Here's how the part is built. I have some questions about the finished solid (model axes, mm). Face numbers are marked on the shaded views. A direction names the side the tool comes from. Coordinates: 2 decimals unless noted, no trailing zeros. Write each loop counter-clockwise with the first axis right and the second up, starting at its lowest first coordinate (ties: lowest second). Pieces come first, ordered by that corner, then holes. Notation, with made-up numbers: (38.5, 9) -> (67.5, 9) arc R27 ccw to (67.5, 47) -> close; hole circle Ø7 at (80, -5.75). An arc over 180 degrees is marked (long way). Put each result on its own line as item: value.
Autodesk Inventor part; units mm, degrees
ref_plane "YZ Plane" through (0, 0, 0) normal (1, 0, 0) x (0, 1, 0)
ref_plane "XZ Plane" through (0, 0, 0) normal (0, 1, 0) x (-1, 0, 0)
ref_plane "XY Plane" through (0, 0, 0) normal (0, 0, 1) x (1, 0, 0)
sketch "Sketch1" plane through (0, 0, 0) normal (0, 0, 1) x (1, 0, 0)
  line L0 (0, 0) -> (60, 0)
  line L1 (60, 0) -> (60, 24)
  line L2 (60, 24) -> (0, 24)
  line L3 (0, 24) -> (0, 0)
  dimension "d0" = 60
  dimension "d1" = 24
extrude "Extrusion1" add sketch "Sketch1" along normal blind 51.8
sketch "Sketch2" plane through (60, 0, 0) normal (1, 0, 0) x (0, 0, -1)
  line L0 (-51.8, 24) -> (-51.8, 0)
  line L1 (0, 0) -> (-51.8, 0)
  line L2 (0, 0) -> (0, 24)
  line L3 (0, 24) -> (-51.8, 24)
  line L4 (-51.8, 14) -> (-18, 14)
  arc A0 (-18, 6) -> (-6, 6) centre (-12, 6) ccw
  line L5 (-18, 6) -> (-18, 14)
  line L6 (-6, 6) -> (-6, 19)
  line L7 (-6, 19) -> (0, 19)
  dimension "d5" = 10
  dimension "d6" = 18
  dimension "d7" = 12
  dimension "d8" = 5
  dimension "d9" = 6
extrude "Extrusion2" cut sketch "Sketch2" against normal blind 60 contours L4 L5 A0 L1 L0 | L2 L1 A0 L6 L7
sketch "Sketch3" plane through (0, 0, 51.8) normal (0, 0, 1) x (1, 0, 0)
  line L0 (60, 0) -> (0, 0)
  line L1 (55, 19) -> (55, 0)
  line L2 (55, 0) -> (60, 0)
  line L3 (60, 0) -> (60, 19)
  line L4 (5, 19) -> (5, 0)
  line L5 (5, 0) -> (0, 0)
  line L6 (0, 0) -> (0, 19)
  line L7 (60, 19) -> (0, 19)
  line L8 (0, 24) -> (60, 24)
  line L9 (0, 0) -> (0, 24)
  line L10 (60, 24) -> (60, 0)
  line L11 (0, 19) -> (5, 19)
  line L12 (55, 19) -> (60, 19)
  point P0 (0, 14)
  point P1 (60, 14)
  dimension "d16" = 5
  dimension "d17" = 5
extrude "Extrusion3" cut sketch "Sketch3" against normal blind 52 contours L0 L1 L7 L3 | L0 L6 L7 L4
chamfer "Chamfer1" distance 10 angle 15 1 edges at (30, 24, 51.8) measured on face at (21.6667, 22.3333, 51.8)
sketch "Sketch5" plane through (55, 19, 6) normal (0, 0, -1) x (-1, 0, 0)
  line L0 (0, 0) -> (0, -13)
  line L1 (-5, 5) -> (55, 5)
  point P0 (55, -19)
  point P1 (6, -9)
  point P2 (44, -9)
  dimension "d35" = 38
  dimension "d36" = 6
  dimension "d37" = 14
  dimension "d38" = 14
hole "Hole2" at (49, 10, 6) at (11, 10, 6) direction (0, 0, 1) diameter 4.917 depth 10 tip angle 118
chamfer "Chamfer2" distance 0.5 angle 45 2 edges at (11, 7.5415, 6) (49, 7.5415, 6)
properties part number "TETO DA CABINE(15)" material "Carbon Steel"
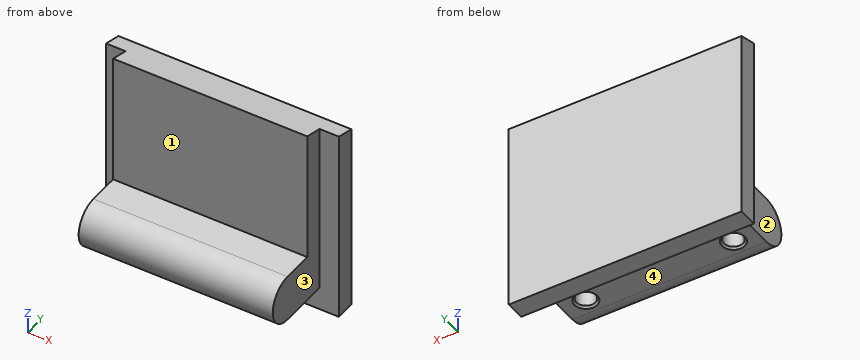
Item 1: Which directions (+Z, -Z, +X, -X, +Y, -Y) give clear straight access to the entire face, cutting with the end or side of a thin tool? Please do the marked faces 1, 2, 3 and 4.
Output:
face 1: +Z, +X, -X, -Y
face 2: +Z, -Z, -X, -Y
face 3: +Z, -Z, +X, -Y
face 4: -Z, +X, -X, -Y
Item 2: For P1, Ø1.5, axis at y = 14, z = 15, coming from the +X side; P2, Ø6.5, axis at x = 19.5, y = 14, coming from the -Z side; P3, Ø25, axis at x = 38, z = 34.5, coming from the -Y side; P4, Ø1, axis at y = 13, z = 32.5, coming from the +X side, each with a flat end and sliding along its axis, tell me the tip position at first contact or that it passes through.
Output:
P1: stops at x = 55
P2: stops at z = 6
P3: stops at y = 14
P4: passes through
Item 3: Please list where these lines run through material, in increasing order: line 1 along X through (y, z) = (10, 12.75); line 2 along Y through (x, z) = (49, 12); line 3 along Y through (x, z) = (51, 19). Write a range as from..to.
Output:
line 1: x = 5..8.54, 13.46..46.54, 51.46..55
line 2: y = 0..7.54, 12.46..24
line 3: y = 14..24
Item 4: Imagine slicing it at C-C on y = 2.5. Write out the boundary of the cut face in (x, z).
Output:
outline: (5, 7.13) -> (55, 7.13) -> (55, 16.87) -> (5, 16.87) -> close
Item 5: Imagine slicing it at A-A on z = 24.5. Write out the boundary of the cut face in (x, y), then the cut area to 3 significant figures.
Output:
outline: (0, 19) -> (5, 19) -> (5, 14) -> (55, 14) -> (55, 19) -> (60, 19) -> (60, 24) -> (0, 24) -> close
area: 550 mm²
